Solid Edge part; units mm, degrees
sketch "Sketch1" plane through (0, 0, 0) normal (0, 0, 1) x (1, 0, 0)
  circle A0 centre (0, 0) radius 70
extrude "Protrusion1" add sketch "Sketch1" along normal blind 20
sketch "Sketch2" plane through (0, 0, 20) normal (0, 0, 1) x (1, 0, 0)
  circle A0 centre (0, 0) radius 50
extrude "ExtrudedProtrusion_2" add sketch "Sketch2" along normal blind 20
sketch "Sketch3" plane through (0, 0, 40) normal (0, 0, 1) x (1, 0, 0)
  circle A0 centre (0, 0) radius 35
extrude "ExtrudedProtrusion_3" add sketch "Sketch3" along normal blind 70
sketch "Sketch4" plane through (0, 0, 110) normal (0, 0, 1) x (1, 0, 0)
  circle A0 centre (0.7844, 0) radius 25
extrude "ExtrudedCutout_1" cut sketch "Sketch4" against normal blind 217.955
sketch "Sketch5" plane through (0, 0, 20) normal (0, 0, 1) x (1, 0, 0)
  circle A0 centre (-62.2319, 0) radius 5
  circle A1 centre (61.4475, 0) radius 5
  circle A2 centre (2.6148, -61.3167) radius 5
  circle A3 centre (0.2615, 62.1012) radius 5
extrude "ExtrudedCutout_2" cut sketch "Sketch5" against normal blind 134.0931
The listing builds one solid part. Answer for the finished solid, in the listing's coordinates (mm). A direction names the side the tool comes from. Coordinates: 2 decimals unless noted, no trailing zeros. Order: outer loops, then holes, each group sorted by start corner. A loop starts at its lowest first (then second) coordinate and runs counter-clockwise, first axis right, second up. Notation, with made-up numbers: M 69,65 L 113,65 A25 cw 113,102 Z; hole C 7,7.25 d2. An arc over 180 degrees is marked long. Answer as a JSON object with one key per item and string values. Group by question number.
1. Determine the mould class of faces 3 (the cylindrical face through (1.531, -66.198, 10.14)), 4 (the cylindrical face through (-28, 21, 75)), 5 (the flat face through (-1, -30, 0)) for opening direction Y: released by +Y, released by -Y, zero draft, split by the parting line, or undercut.
2. Flat-ended cylindrical pins translate along their axes: P1, Ø12, axis at x = 32, z = 18, coming from the +Y side; P2, Ø12, axis at x = 21.5, z = 68, coming from the +Y side; P3, Ø9, axis at x = -62.23, y = 0, coming from the +Z side; P4, Ø12, axis at y = 4.5, z = 55, coming from the +X side. Find the tip coordinate at first contact, or state that the pin passes through.
3. Section C-C on y = 21 is taken. Write down the section's boundary in (x, z).
4. Section A-A on y = 0 is taken. Write down the section's boundary in (x, z), then the cut area to 3 significant figures.
5. Section B-B on x = 0 is taken. Write down the section's boundary in (y, z).
6. A tool of negligible diameter and unlimited length cuts with its end or side. For faces 1 (the cylindrical face through (47.69, -15.02, 29.86)), 2 (the cylindrical face through (66.217, 1.502, 10.14)), from which of +Z, -Z, +X, -X, +Y, -Y can it reach the whole face along a straight path? Write none if from no direction.
7. Section D-D on x = -14.5 is taken. Write down the section's boundary in (y, z).
8. Straight lines are drawn through the part: line 1 (Y direction, x = -3.5, z = 7); line 2 (Z direction, x = 25, y = 38.5); line 3 (Z direction, x = -6.5, y = -61). For each, find the intervals that lie inside material, in ascending order.
Values follow:
{
 "1": {"face 3": "undercut", "face 4": "split by the parting line", "face 5": "zero draft"},
 "2": {"P1": "y = 64.99", "P2": "y = 31.38", "P3": "through", "P4": "x = 35"},
 "3": {"outline": "M -66.78,0 L -12.78,0 L -12.78,110 L -28,110 L -28,40 L -45.38,40 L -45.38,20 L -66.78,20 Z; M 14.35,0 L 66.78,0 L 66.78,20 L 45.38,20 L 45.38,40 L 28,40 L 28,110 L 14.35,110 Z"},
 "4": {"outline": "M -70,0 L -67.23,0 L -67.23,20 L -70,20 Z; M -57.23,0 L -24.22,0 L -24.22,110 L -35,110 L -35,40 L -50,40 L -50,20 L -57.23,20 Z; M 25.78,0 L 56.45,0 L 56.45,20 L 50,20 L 50,40 L 35,40 L 35,110 L 25.78,110 Z; M 66.45,0 L 70,0 L 70,20 L 66.45,20 Z", "area": "3,800 mm2"},
 "5": {"outline": "M -70,0 L -65.58,0 L -65.58,20 L -70,20 Z; M -57.05,0 L -24.99,0 L -24.99,110 L -35,110 L -35,40 L -50,40 L -50,20 L -57.05,20 Z; M 24.99,0 L 57.11,0 L 57.11,20 L 50,20 L 50,40 L 35,40 L 35,110 L 24.99,110 Z; M 67.09,0 L 70,0 L 70,20 L 67.09,20 Z"},
 "6": {"face 1": "+Z", "face 2": "+Z, -Z"},
 "7": {"outline": "M -68.48,0 L -19.78,0 L -19.78,110 L -31.86,110 L -31.86,40 L -47.85,40 L -47.85,20 L -68.48,20 Z; M 19.78,0 L 68.48,0 L 68.48,20 L 47.85,20 L 47.85,40 L 31.86,40 L 31.86,110 L 19.78,110 Z"},
 "8": {"line 1": "-69.91 to -24.63, 24.63 to 58.81, 65.4 to 69.91", "line 2": "0 to 40", "line 3": "0 to 20"}
}
